Input: part model. Units: mm. Frame: model coordinates. Face numbers are marked on the shaded views. A direction names the side the tool comes from. Coordinates: 2 decimals unless noted, no trailing zeros. Loops run counter-clockwise (first coordinate to the right, second up) from the corner with the lowest first, then second, coordinate; pieces in that order, holes last.
```python
from build123d import *

# Parameters (mm, degrees)
F1_DEPTH = 1.1938
F2_R     = 1.5
F3_DEPTH = 1.1948
F4_W     = 5
F4_H     = 47.6
F4_H_2   = 38.6
F5_DEPTH = 8.5
F6_W     = 35.585186
F6_H     = 8.839631
F7_DEPTH = 0.0254


with BuildPart() as f1:
    # F0 (on Top) → F1 (new body)
    with BuildSketch(Plane.XY):
        with BuildLine():
            Line((-13.97, -40.64), (13.97, -40.64))
            ThreePointArc((13.97, -40.64), (22.950256, -36.920256), (26.67, -27.94))
            Line((26.67, -27.94), (26.67, 27.94))
            ThreePointArc((26.67, 27.94), (22.950256, 36.920256), (13.97, 40.64))
            Line((13.97, 40.64), (-13.97, 40.64))
            ThreePointArc((-13.97, 40.64), (-22.950256, 36.920256), (-26.67, 27.94))
            Line((-26.67, 27.94), (-26.67, -27.94))
            ThreePointArc((-26.67, -27.94), (-22.950256, -36.920256), (-13.97, -40.64))
        make_face()
    extrude(amount=F1_DEPTH)

    # F2 (on face) → F3 (cut, through all)
    with BuildSketch(Plane.XY.offset(1.1938)):
        with Locations((-23.5, 27.5)):
            Circle(F2_R)
        with Locations((23.5, 27.5)):
            Circle(F2_R)
        with Locations((-23.5, -27.5)):
            Circle(F2_R)
        with Locations((23.5, -26.5)):
            Circle(F2_R)
    extrude(amount=-F3_DEPTH, mode=Mode.SUBTRACT)

    # F4 (on face) → F5 (join)
    with BuildSketch(Plane.XY.offset(1.1938)):
        with Locations((-23.17, 0.5)):
            Rectangle(F4_W, F4_H)
        with Locations((23.17, 5)):
            Rectangle(F4_W, F4_H_2)
    extrude(amount=F5_DEPTH)

    # F6 (on face) → F7 (join)
    with BuildSketch(Plane.XY.offset(1.1938)):
        with Locations((1e-06, 31.618683)):
            Rectangle(F6_W, F6_H)
    extrude(amount=F7_DEPTH)


solid = f1.part
```
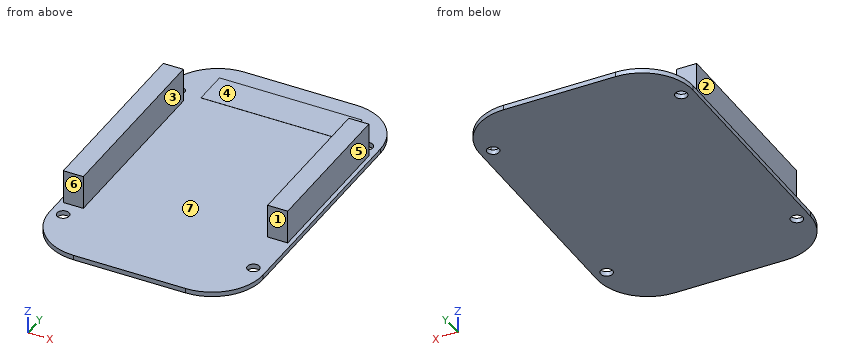
Item 1: Line query: L1, parallel to X at y = -12.5, z = 5; L2, parallel to Y at x = 23.5, z = 0.7; L3, parallel to Z at x = 8, y = -29.5. Output: solid intervals per line, ascending.
Result:
L1: x = -25.67 to -20.67, 20.67 to 25.67
L2: y = -36.33 to -28, -25 to 26, 29 to 36.33
L3: z = 0 to 1.19
Item 2: Reachability of the marked faces 1, 2, 3 and 4 from +Z, -Z, +X, -X, +Y, -Y: full face, straight path, thin tool, end or side. Return the list, or none.
Result:
face 1: +Z, +X, -Y
face 2: +Z, -X, +Y, -Y
face 3: +Z, +Y, -Y
face 4: +Z, +X, -X, +Y, -Y
Item 3: Section query A-A (z = 7). Output: boundary loops of the cut face in (x, y), then the cut area to 3 significant figures.
Result:
outline: (-25.67, -23.3) - (-20.67, -23.3) - (-20.67, 24.3) - (-25.67, 24.3) - close; (20.67, -14.3) - (25.67, -14.3) - (25.67, 24.3) - (20.67, 24.3) - close
area: 431 mm2
Item 4: Mould query, pull axis X, two halves, no side actions, for the marked faces 5, 6 and 7. Classes: +X half, -X half, draft (parallel to the pull), parting line (faces both ways), or undercut.
Result:
face 5: +X half
face 6: draft
face 7: undercut
Item 5: Section query B-B (x = 23.5). Output: boundary loops of the cut face in (y, z).
Result:
outline: (-36.33, 0) - (-28, 0) - (-28, 1.19) - (-36.33, 1.19) - close; (-25, 0) - (26, 0) - (26, 1.19) - (24.3, 1.19) - (24.3, 9.69) - (-14.3, 9.69) - (-14.3, 1.19) - (-25, 1.19) - close; (29, 0) - (36.33, 0) - (36.33, 1.19) - (29, 1.19) - close
Item 6: Contact query for flat-ended pins moving along their axis: P1, Ø3, axis at x = 7, z = 3.5, coming from the +Y side; P2, Ø1.5, axis at y = 32.5, z = 1.5, coming from the +X side; P3, Ø4, axis at x = -23, z = 5, coming from the +Y side; P4, Ø4, axis at y = 9.5, z = 5, coming from the +X side. Output: stop coordinate, or through.
Result:
P1: passes through
P2: stops at x = 26.06
P3: stops at y = 24.3
P4: stops at x = 25.67
Item 7: Section query D-D (x = -23.5). Output: boundary loops of the cut face in (y, z), then the cut area to 3 significant figures.
Result:
outline: (-36.33, 0) - (-29, 0) - (-29, 1.19) - (-36.33, 1.19) - close; (-26, 0) - (26, 0) - (26, 1.19) - (24.3, 1.19) - (24.3, 9.69) - (-23.3, 9.69) - (-23.3, 1.19) - (-26, 1.19) - close; (29, 0) - (36.33, 0) - (36.33, 1.19) - (29, 1.19) - close
area: 484 mm2
